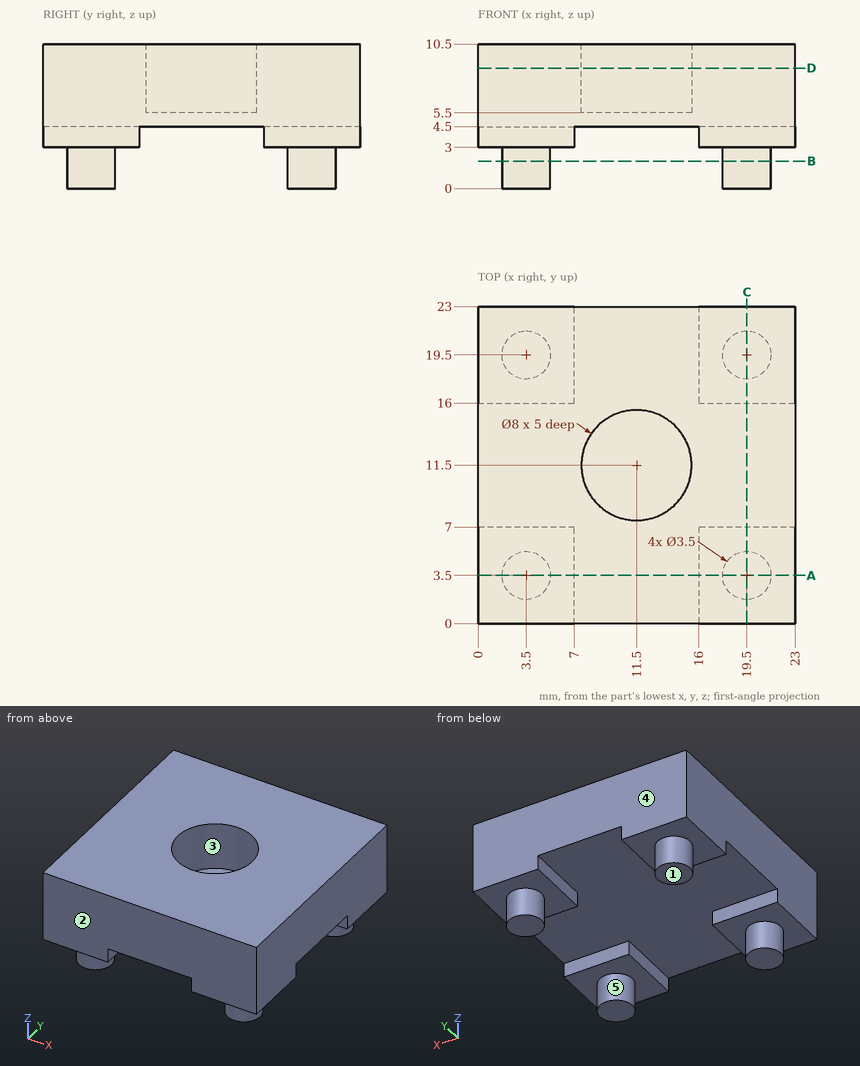
Geometry: see drawing. Coordinates: mm, zero at the bounding-box minimum. A direction names the side the tool comes from. Round coordinates to 2 decimals unless told otherwise and drop trailing zeros. Write each loop counter-clockwise with the first axis right and the second up, starting at its lowest first coordinate (ties: lowest second). Pieces come first, ordered by that corner, then holes.
Item 1: Section query D-D (z = 8.75). Return loops of the section in (x, y), plus the area to 3 significant figures.
Item 2: Pin query (flat end, axial travel): P1, Ø1.5, axis at x = 20.5, z = 1.5, coming from the +Y side. Return the tip coordinate at first contact, or that it passes through.
Item 3: Material intervals for L1, parallel to Y at x = 11.5, z = 9.05; L2, parallel to Z at x = 9.5, y = 17.75; L3, parallel to Y at x = 9.25, z = 10, sorted ascending.
Item 4: Mould query, pull axis Y, two halves, no side actions, for the marked faces 1, 2 and 3. Classes: +Y half, -Y half, draft (parallel to the pull), parting line (faces both ways), or undercut.
Item 5: Set-up query: the marked faces 4 and 5. Return all of +Z, -Z, +X, -X, +Y, -Y with unobstructed straight access to the full face (end or side cutting, diameter ignored); none if empty.
Item 6: Section query B-B (z = 2). Return loops of the section in (x, y).
Item 7: Section query A-A (y = 3.5). Return loops of the section in (x, z), plus the area to 3 significant figures.
Completed:
1. outline: (0, 0) - (23, 0) - (23, 23) - (0, 23) - close; hole circle Ø8 at (11.5, 11.5)
1. area: 479 mm2
2. P1: stops at y = 21.23
3. L1: y = 0 to 7.5, 15.5 to 23
3. L2: z = 4.5 to 10.5
3. L3: y = 0 to 8.19, 14.81 to 23
4. face 1: draft
4. face 2: -Y half
4. face 3: undercut
5. face 4: +Z, -Z, +X, -X, +Y
5. face 5: -Z
6. outline: circle Ø3.5 at (3.5, 3.5); circle Ø3.5 at (3.5, 19.5); circle Ø3.5 at (19.5, 3.5); circle Ø3.5 at (19.5, 19.5)
7. outline: (0, 3) - (1.75, 3) - (1.75, 0) - (5.25, 0) - (5.25, 3) - (7, 3) - (7, 4.5) - (16, 4.5) - (16, 3) - (17.75, 3) - (17.75, 0) - (21.25, 0) - (21.25, 3) - (23, 3) - (23, 10.5) - (0, 10.5) - close
7. area: 180 mm2
